Here's the drawing with two shaded views (mm, measured from the low corner). I have some questions. Give positions to 0.01 mm unless a question says otherwise; leave off trailing zeros. Order: outer loops, then holes, each group sorted by start corner. A loop starts at its lowest first (then second) coordinate and runs counter-clockwise, first axis right, second up. Notation, with made-up numbers: M -37.5,-31 L -18.5,-31 A27 cw -18.5,2 Z; hole C 55,-11.5 d9. An arc over 180 degrees is marked long. One line per question, with ' | ' between items. Start each with the question number.
1) Please list where this line runs through material, in increasing order: line 1 along X through (y, z) = (26, 38.5). Write a range as [from, to].
2) I'm going to push flat-ended pins straight in: pin 1 Ø3 at (x, z) = (11.5, 69.5) entering from +Y; pin 2 Ø1.3 at (x, z) = (7.5, 65.5) entering from +Y. Where does each tip first touch, or does it pass through?
3) If we section it at A-A, the plane y = 35.5: Please give me the cut outline in (x, z).
4) Thinking about a two-plate mould opening in Z: for the marked faces 1, 2 and 3, which applies, +Z half, -Z half, draft (parallel to the pull), parting line (faces both ways), or undercut?
5) If we section it at B-B, the plane z = 70: Please give me the cut outline in (x, y).
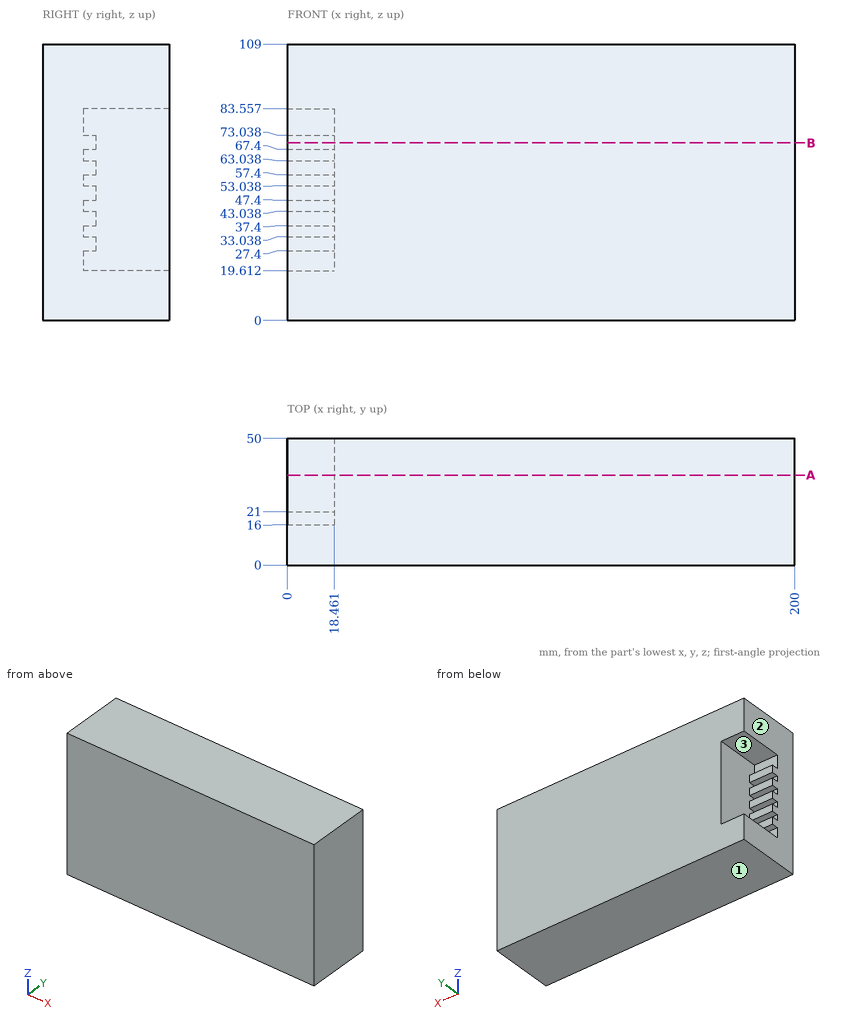
Results found:
1) line 1: x = [18.46, 200]
2) pin 1: stops at y = 21 | pin 2: stops at y = 16
3) outline: M 0,0 L 200,0 L 200,109 L 0,109 L 0,83.56 L 18.46,83.56 L 18.46,19.61 L 0,19.61 Z
4) face 1: -Z half | face 2: draft | face 3: undercut
5) outline: M 0,0 L 200,0 L 200,50 L 18.46,50 L 18.46,21 L 0,21 Z
